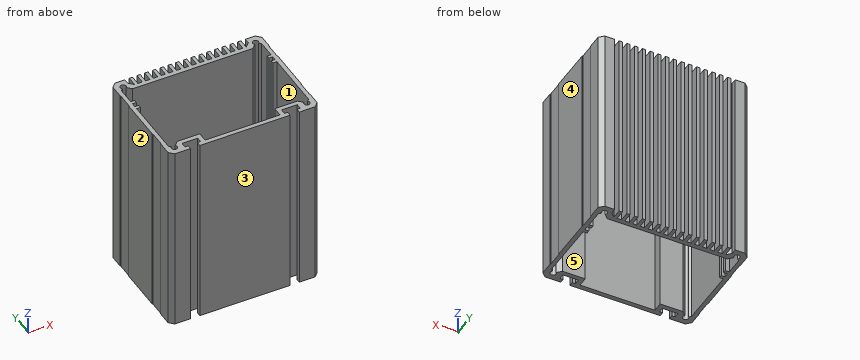
```python
from build123d import *

# Parameters (mm, degrees)
BOSS_EXTRUDE1_DEPTH = 87.4395


with BuildPart() as part:
    # Sketch1 → Boss-Extrude1 (new body)
    with BuildSketch(Plane.XY.offset(12.5605)):
        Polygon((-54.188249545, 1.80757214), (-54.188249545, -0.19242786), (-13.388249545, -0.19242786), (-13.388249545, 1.80757214), (-14.838249545, 1.80757214), (-14.838249545, 4.30757214), (-7.738249545, 4.30757214), (-7.738249545, 1.80757214), (-9.188249545, 1.80757214), (-9.188249545, -0.19242786), (-2.088249216, -0.19242786), (-0.088249545, 1.807571812), (-0.088249545, 8.007572024), (-0.288249545, 8.207572024), (-0.288249545, 15.00757214), (-0.088249545, 15.20757214), (-0.088249545, 35.20757214), (-0.288249545, 35.40757214), (-0.288249545, 42.207572024), (-0.088249545, 42.407572024), (-0.088249545, 48.607572237), (-2.088249448, 50.60757214), (-6.538249545, 50.60757214), (-6.538249545, 48.10757214), (-8.538249545, 46.10757214), (-8.538249545, 50.60757214), (-10.038249545, 50.60757214), (-10.038249545, 46.10757214), (-12.038249545, 46.10757214), (-12.038249545, 50.60757214), (-13.538249545, 50.60757214), (-13.538249545, 46.10757214), (-15.538249545, 46.10757214), (-15.538249545, 50.60757214), (-17.038249545, 50.60757214), (-17.038249545, 46.10757214), (-19.038249545, 46.10757214), (-19.038249545, 50.60757214), (-20.538249545, 50.60757214), (-20.538249545, 46.10757214), (-22.538249545, 46.10757214), (-22.538249545, 50.60757214), (-24.038249545, 50.60757214), (-24.038249545, 46.10757214), (-26.038249545, 46.10757214), (-26.038249545, 50.60757214), (-27.538249545, 50.60757214), (-27.538249545, 46.10757214), (-29.538249545, 46.10757214), (-29.538249545, 50.60757214), (-31.038249545, 50.60757214), (-31.038249545, 46.10757214), (-33.038249545, 46.10757214), (-33.038249545, 50.60757214), (-34.538249545, 50.60757214), (-34.538249545, 46.10757214), (-36.538249545, 46.10757214), (-36.538249545, 50.60757214), (-38.038249545, 50.60757214), (-38.038249545, 46.10757214), (-40.038249545, 46.10757214), (-40.038249545, 50.60757214), (-41.538249545, 50.60757214), (-41.538249545, 46.10757214), (-43.538249545, 46.10757214), (-43.538249545, 50.60757214), (-45.038249545, 50.60757214), (-45.038249545, 46.10757214), (-47.038249545, 46.10757214), (-47.038249545, 50.60757214), (-48.538249545, 50.60757214), (-48.538249545, 46.10757214), (-50.538249545, 46.10757214), (-50.538249545, 50.60757214), (-52.038249545, 50.60757214), (-52.038249545, 46.10757214), (-54.038249545, 46.10757214), (-54.038249545, 50.60757214), (-55.538249545, 50.60757214), (-55.538249545, 46.10757214), (-57.538249545, 46.10757214), (-57.538249545, 50.60757214), (-59.038249545, 50.60757214), (-59.038249545, 46.10757214), (-61.038249545, 48.10757214), (-61.038249545, 50.60757214), (-65.488249642, 50.60757214), (-67.488249545, 48.607572237), (-67.488249545, 42.407572024), (-67.288249545, 42.207572024), (-67.288249545, 35.40757214), (-67.488249545, 35.20757214), (-67.488249545, 15.20757214), (-67.288249545, 15.00757214), (-67.288249545, 8.207572024), (-67.488249545, 8.007572024), (-67.488249545, 1.807571812), (-65.488249874, -0.19242786), (-58.388249545, -0.19242786), (-58.388249545, 1.80757214), (-59.838249545, 1.80757214), (-59.838249545, 4.30757214), (-52.738249545, 4.30757214), (-52.738249545, 1.80757214), align=None)
        with BuildLine():
            Line((-2.088249545, 32.20757214), (-2.088249545, 5.294016009))
            Line((-2.088249545, 5.294016009), (-2.963249358, 4.419016196))
            ThreePointArc((-2.963249358, 4.419016196), (-3.838249708, 2.15757214), (-4.713249491, 4.419016416))
            Line((-4.713249491, 4.419016416), (-6.601805216, 6.30757214))
            Line((-6.601805216, 6.30757214), (-16.838249545, 6.30757214))
            Line((-16.838249545, 6.30757214), (-16.838249545, 1.807572024))
            Line((-16.838249545, 1.807572024), (-50.738249545, 1.807572024))
            Line((-50.738249545, 1.807572024), (-50.738249545, 6.30757214))
            Line((-50.738249545, 6.30757214), (-60.974693874, 6.30757214))
            Line((-60.974693874, 6.30757214), (-62.863249599, 4.419016416))
            ThreePointArc((-62.863249599, 4.419016416), (-63.738249382, 2.15757214), (-64.613249732, 4.419016196))
            Line((-64.613249732, 4.419016196), (-65.488249545, 5.294016009))
            Line((-65.488249545, 5.294016009), (-65.488249545, 32.20757214))
            Line((-65.488249545, 32.20757214), (-63.738249545, 32.20757214))
            Line((-63.738249545, 32.20757214), (-63.738249545, 33.70757214))
            Line((-63.738249545, 33.70757214), (-65.488249545, 33.70757214))
            Line((-65.488249545, 33.70757214), (-65.488249545, 35.70757214))
            Line((-65.488249545, 35.70757214), (-63.738249545, 35.70757214))
            Line((-63.738249545, 35.70757214), (-63.738249545, 37.20757214))
            Line((-63.738249545, 37.20757214), (-65.488249545, 37.20757214))
            Line((-65.488249545, 37.20757214), (-65.488249545, 45.121128024))
            Line((-65.488249545, 45.121128024), (-64.613249603, 45.996127967))
            ThreePointArc((-64.613249603, 45.996127967), (-63.738249551, 48.25757214), (-62.863249479, 45.996127974))
            Line((-62.863249479, 45.996127974), (-60.974693645, 44.10757214))
            Line((-60.974693645, 44.10757214), (-6.601805445, 44.10757214))
            Line((-6.601805445, 44.10757214), (-4.713249611, 45.996127974))
            ThreePointArc((-4.713249611, 45.996127974), (-3.838249539, 48.25757214), (-2.963249487, 45.996127967))
            Line((-2.963249487, 45.996127967), (-2.088249545, 45.121128024))
            Line((-2.088249545, 45.121128024), (-2.088249545, 37.20757214))
            Line((-2.088249545, 37.20757214), (-3.838249545, 37.20757214))
            Line((-3.838249545, 37.20757214), (-3.838249545, 35.70757214))
            Line((-3.838249545, 35.70757214), (-2.088249545, 35.70757214))
            Line((-2.088249545, 35.70757214), (-2.088249545, 33.70757214))
            Line((-2.088249545, 33.70757214), (-3.838249545, 33.70757214))
            Line((-3.838249545, 33.70757214), (-3.838249545, 32.20757214))
            Line((-3.838249545, 32.20757214), (-2.088249545, 32.20757214))
        make_face(mode=Mode.SUBTRACT)
    extrude(amount=BOSS_EXTRUDE1_DEPTH)


solid = part.part
```
Input: part model. Units: mm. Frame: model coordinates. Face numbers are marked on the shaded views. A direction names the side the tool comes from. Give positions to 0.01 mm unless a question says otherwise; leave off trailing zeros. Order: outer loops, then holes, each group sorted by start corner. A loop starts at its lowest first (then second) coordinate and runs counter-clockwise, first axis right, second up. Notation, with made-up numbers: M -10,9.25 L 8,9.25 A21 cw 8,40.25 Z; hole C -30,49.25 d6. An arc over 180 degrees is marked long. One line per question, with ' | ' between items. Start each with the question number.
1. Section query B-B (y = 40). Return the cut outline in (x, z).
2. Section query A-A (y = 30). Return the cut outline in (x, z), and give its area (3 significant figures).
3. Access query for the marked faces 1 and 2. Directions: +Z, -Z, +X, -X, +Y, -Y. A direction counts if a zero-diameter tool reaches every point of the face in a straight line with its end or side. Return the directions, or none.
4. Pull-direction query (Y, two-part tool) for the marked faces 3, 4 and 5; classes: released by +Y, released by -Y, zero draft, split by the parting line, or undercut.
5. Material intervals for probe 1 along Y at (x, z) = (-9, 61); probe 2 along X at (y, z) = (20, 46); probe 3 along Y at (x, z) = (-36.5, 27.5), sorted ascending. Write a range as [from, to].
6. First-contact query: pin 1 Ø10 at (x, y) = (-44.5, 8.5) entering from -Z; pin 2 Ø2.5 at (y, z) = (42, 44) entering from +X; pin 3 Ø0.6 at (y, z) = (0.5, 38) entering from +X. Flat tips, straight axial feed; report the tip coordinate or a pass-through.
Here are the results:
1) outline: M -67.29,12.56 L -65.49,12.56 L -65.49,100 L -67.29,100 Z; M -2.09,12.56 L -0.29,12.56 L -0.29,100 L -2.09,100 Z
2) outline: M -67.49,12.56 L -65.49,12.56 L -65.49,100 L -67.49,100 Z; M -2.09,12.56 L -0.09,12.56 L -0.09,100 L -2.09,100 Z | area: 350 mm²
3) face 1: +Z, -Z | face 2: +Z, -Z, -X, +Y, -Y
4) face 3: released by -Y | face 4: zero draft | face 5: undercut
5) probe 1: [-0.19, 1.81], [4.31, 6.31], [44.11, 50.61] | probe 2: [-67.49, -65.49], [-2.09, -0.09] | probe 3: [-0.19, 1.81], [44.11, 46.11]
6) pin 1: through | pin 2: x = -0.09 | pin 3: x = -1.1
